from build123d import *

# Parameters (mm, degrees)
SKETCH_1_W          = 60
SKETCH_1_H          = 125
EXTRUDE_1_DEPTH     = 5
SKETCH_4_R          = 19.5
CUT_EXTRUDE_2_DEPTH = 10
SKETCH_2_R          = 2.5
CUT_EXTRUDE_1_DEPTH = 5


with BuildPart() as part:
    # 스케치1 → 보스-돌출1 (new body)
    with BuildSketch(Plane.XY):
        Rectangle(SKETCH_1_W, SKETCH_1_H)
    extrude(amount=EXTRUDE_1_DEPTH)

    # 스케치4 → 컷-돌출2 (cut)
    with BuildSketch(Plane(origin=(0, 0, 0), x_dir=(-1, 0, 0), z_dir=(0, 0, -1))):
        with Locations((0, 32.5)):
            Circle(SKETCH_4_R)
    extrude(amount=-CUT_EXTRUDE_2_DEPTH, mode=Mode.SUBTRACT)

    # 스케치2 → 컷-돌출1 (cut)
    with BuildSketch(Plane.XY.offset(5)):
        with Locations((23.57, 56.07)):
            Circle(SKETCH_2_R)
        with Locations((23.57, 8.93)):
            Circle(SKETCH_2_R)
        with Locations((-23.57, 8.93)):
            Circle(SKETCH_2_R)
        with Locations((-23.57, 56.07)):
            Circle(SKETCH_2_R)
    extrude(amount=-CUT_EXTRUDE_1_DEPTH, mode=Mode.SUBTRACT)


solid = part.part
Design review of the part built by this model. Coordinates are the model's own, in mm. Round coordinates to 2 decimals unless told otherwise and drop trailing zeros. Write each loop counter-clockwise with the first axis right and the second up, starting at its lowest first coordinate (ties: lowest second). Pieces come first, ordered by that corner, then holes. Notation, with made-up numbers: (-14.5, 51.5) - (26.5, 51.5) arc R35 ccw to (26.5, 87.5) - close; hole circle Ø9 at (-12, -21). An arc over 180 degrees is marked (long way). Use a Markdown table: item, result. Add a question column.
1. We need section D-D (z = 2.1). State the section outline as (x, y) points, then the cut area to 3 significant figures.
2. We need section C-C (x = -23.57). State the section outline as (y, z) points, then the cut area to 3 significant figures.
3. We need section A-A (x = 0). State the section outline as (y, z) points, then the cut area to 3 significant figures.
4. Mouldability with a two-part tool opening along X and no side actions: class faces 1 (the face through (0, 1, 5)), 2 (the face through (-23.9, 11.41, 2.54)), 3 (the face through (30, -1, 2)) as +X half, -X half, draft (parallel to the pull), parting line (faces both ways), or undercut.
5. Wall thickness on probe 1 along Y at (x, z) = (23.57, 2.75); probe 2 along X at (y, z) = (27.5, 2.3); probe 3 along Y at (x, z) = (5.5, 3.5): over which ranges is each line inside the solid? List them lowest first.
6. We need section B-B (y = 8.93). State the section outline as (x, z) points, then the cut area to 3 significant figures.
Output:
| question | item | result |
|---|---|---|
| 1 | outline | (-30, -62.5) - (30, -62.5) - (30, 62.5) - (-30, 62.5) - close; hole circle Ø5 at (-23.57, 8.93); hole circle Ø5 at (-23.57, 56.07); hole circle Ø39 at (0, 32.5); hole circle Ø5 at (23.57, 8.93); hole circle Ø5 at (23.57, 56.07) |
| 1 | area | 6,230 mm2 |
| 2 | outline | (-62.5, 0) - (6.43, 0) - (6.43, 5) - (-62.5, 5) - close; (11.43, 0) - (53.57, 0) - (53.57, 5) - (11.43, 5) - close; (58.57, 0) - (62.5, 0) - (62.5, 5) - (58.57, 5) - close |
| 2 | area | 575 mm2 |
| 3 | outline | (-62.5, 0) - (13, 0) - (13, 5) - (-62.5, 5) - close; (52, 0) - (62.5, 0) - (62.5, 5) - (52, 5) - close |
| 3 | area | 430 mm2 |
| 4 | face 1 | draft |
| 4 | face 2 | undercut |
| 4 | face 3 | +X half |
| 5 | probe 1 | y = -62.5 to 6.43, 11.43 to 53.57, 58.57 to 62.5 |
| 5 | probe 2 | x = -30 to -18.85, 18.85 to 30 |
| 5 | probe 3 | y = -62.5 to 13.79, 51.21 to 62.5 |
| 6 | outline | (-30, 0) - (-26.07, 0) - (-26.07, 5) - (-30, 5) - close; (-21.07, 0) - (21.07, 0) - (21.07, 5) - (-21.07, 5) - close; (26.07, 0) - (30, 0) - (30, 5) - (26.07, 5) - close |
| 6 | area | 250 mm2 |
